```python
from build123d import *

# Parameters (mm, degrees)
EXTRUDE_1_DEPTH     = 2
EXTRUDE_2_DEPTH     = 1.2
SKETCH_4_R          = 1.55
EXTRUDE_3_DEPTH     = 4
EXTRUDE_START       = 3
SKETCH_4_3_R        = 1.55
EXTRUDE_4_DEPTH     = 4
FILLET_1_R          = 3
SKETCH_5_W          = 3.5
SKETCH_5_H          = 2.5
EXTRUDE_5_DEPTH     = 59.375418161
SKETCH_9_W          = 7
SKETCH_9_H          = 4
CUT_EXTRUDE_3_DEPTH = 2
OTHER_START         = -350.004341608
OTHER_1_OUTLINE_W   = 1.5
OTHER_1_OUTLINE_H   = 5.2
OTHER_1_OUTLINE_W_2 = 5.2
OTHER_1_OUTLINE_H_2 = 1.5
OTHER_1_DEPTH       = 1.2
SKETCH_10_R         = 3.4
SKETCH_10_R_2       = 1.4
EXTRUDE_6_DEPTH     = 13.8
EXTRUDE_7_DEPTH     = 2.4
CHAMFER_1_SIZE2     = 1.219331471
CHAMFER_1_SIZE      = 2.5
EXTRUDE_9_DEPTH     = 15.389983971
SKETCH_15_R         = 1.5
CUT_EXTRUDE_4_DEPTH = 407.679532375
FILLET_2_R          = 3
SKETCH_16_R         = 3
CUT_EXTRUDE_5_DEPTH = 408.922716855


# Read off the part's stored shape, not the designer's step: Отступ1
# Some blends are built 0.0001 mm under size
with BuildPart() as part:
    # Эскиз2 → Бобышка-Вытянуть1 (new body)
    with BuildSketch(Plane.XY.offset(0.1)):
        Polygon((-376.904341608, -14.952219826), (-393.804341608, -14.952219826), (-393.804341608, 44.423198335), (-348.804341608, 44.423198335), (-348.804341608, -19.952219826), (-376.904341608, -19.952219826), align=None)
    extrude(amount=EXTRUDE_1_DEPTH)

    # Эскиз3 → Бобышка-Вытянуть2 (add)
    with BuildSketch(Plane(origin=(-348.804341608, 0, 0), x_dir=(0, 0, -1), z_dir=(1, 0, 0))):
        with BuildLine():
            Line((-0.1, -19.952219826), (-0.1, 45.823198335))
            Line((-0.1, 45.823198335), (-58.7849644, 45.823198335))
            ThreePointArc((-58.7849644, 45.823198335), (-79.43775717, 37.268531468), (-87.992424037, 16.615738698))
            Line((-87.992424037, 16.615738698), (-87.992424037, -19.952219826))
            Line((-87.992424037, -19.952219826), (-0.1, -19.952219826))
        make_face()
    extrude(amount=-EXTRUDE_2_DEPTH)

    # Эскиз4 → Бобышка-Вытянуть3 (add)
    with BuildSketch(Plane(origin=(0, -17.952219826, 0), x_dir=(1, 0, 0), z_dir=(0, 1, 0))):
        with BuildLine():
            Line((-357.604341608, -2.1), (-357.604341608, -5.7))
            ThreePointArc((-357.604341608, -5.7), (-356.608504664, -8.104163056), (-354.204341608, -9.1))
            Line((-354.204341608, -9.1), (-350.004341608, -9.1))
            Line((-350.004341608, -9.1), (-350.004341608, -2.1))
            Line((-350.004341608, -2.1), (-357.604341608, -2.1))
        make_face()
        with Locations(Location((-354.204341608, -5.7, 0), (0, 0, 270))):
            Circle(SKETCH_4_R, mode=Mode.SUBTRACT)
    extrude(amount=EXTRUDE_3_DEPTH)

    # Эскиз4<3> → Бобышка-Вытянуть4 (add)
    with BuildSketch(Plane(origin=(0, -17.952219826, 0), x_dir=(1, 0, 0), z_dir=(0, 1, 0)).offset(EXTRUDE_START)):
        with BuildLine():
            Line((-390.304341608, -5.7), (-390.304341608, -2.1))
            Line((-390.304341608, -2.1), (-381.365657691, -2.1))
            Line((-381.365657691, -2.1), (-383.84844185, -7.190461899))
            ThreePointArc((-383.84844185, -7.190461899), (-387.669175192, -9.01285822), (-390.304341608, -5.7))
        make_face()
        with Locations(Location((-386.904341608, -5.7, 0), (0, 0, 180))):
            Circle(SKETCH_4_3_R, mode=Mode.SUBTRACT)
    extrude(amount=EXTRUDE_4_DEPTH)

    # Скругление1
    fillet_1_edges = [part.edges().sort_by_distance(p)[0] for p in [
        (-350.004341608, -18.952219826, 2.1),
        (-350.004341608, 15.235489254, 2.1),
    ]]
    fillet(fillet_1_edges, radius=FILLET_1_R)

    # Эскиз5 → Бобышка-Вытянуть5 (add)
    with BuildSketch(Plane(origin=(0, 44.423198335, 0), x_dir=(1, 0, 0), z_dir=(0, 1, 0))):
        with Locations((-392.054341608, -3.35)):
            Rectangle(SKETCH_5_W, SKETCH_5_H)
    extrude(amount=-EXTRUDE_5_DEPTH)

    # Эскиз9 → Вырез-Вытянуть3 (cut)
    with BuildSketch(Plane(origin=(0, 0, 0.1), x_dir=(-1, 0, 0), z_dir=(0, 0, -1))):
        with Locations((385.390488384, 40.423198335)):
            Rectangle(SKETCH_9_W, SKETCH_9_H)
    extrude(amount=-CUT_EXTRUDE_3_DEPTH, mode=Mode.SUBTRACT)

    # Отступ1 outline → Отступ1 (cut)
    with BuildSketch(Plane.YZ.offset(OTHER_START)):
        with Locations((42.673198335, 13.546937644)):
            Rectangle(OTHER_1_OUTLINE_W, OTHER_1_OUTLINE_H)
        with Locations((42.673198335, 36.546937644)):
            Rectangle(OTHER_1_OUTLINE_W, OTHER_1_OUTLINE_H)
        Polygon((41.843105902, 62.072434127), (41.984560077, 56.874358452), (43.484004983, 56.915162541), (43.342550808, 62.113238216), align=None)
        Polygon((31.397725301, 79.490528515), (35.298941914, 76.052431812), (36.290700579, 77.177782758), (32.389483966, 80.615879461), align=None)
        with Locations((13.847780174, 84.842424037)):
            Rectangle(OTHER_1_OUTLINE_W_2, OTHER_1_OUTLINE_H_2)
        with Locations((-9.152219826, 84.842424037)):
            Rectangle(OTHER_1_OUTLINE_W_2, OTHER_1_OUTLINE_H_2)
    extrude(amount=OTHER_1_DEPTH, mode=Mode.SUBTRACT)

    # Эскиз10 → Бобышка-Вытянуть6 (add)
    # profile 1 of 2: a face of its own
    with BuildSketch(Plane.ZY.offset(350.004341608)):
        with Locations(Location((57.85, 36.323198334, 0), (0, 0, 180))):
            Circle(SKETCH_10_R)
        with Locations(Location((57.85, 36.323198334, 0), (0, 0, 180))):
            Circle(SKETCH_10_R_2, mode=Mode.SUBTRACT)
    # profile 2 of 2: a face of its own
    with BuildSketch(Plane.ZY.offset(350.004341608)):
        with Locations(Location((17.35, 36.323198334, 0), (0, 0, 180))):
            Circle(SKETCH_10_R)
        with Locations(Location((17.35, 36.323198334, 0), (0, 0, 180))):
            Circle(SKETCH_10_R_2, mode=Mode.SUBTRACT)
    extrude(amount=EXTRUDE_6_DEPTH)

    # Эскиз12 → Бобышка-Вытянуть7 (add)
    with BuildSketch(Plane.ZY.offset(350.004341608)):
        with BuildLine():
            Line((77.792424037, 16.615738698), (77.792424037, -19.952219826))
            Line((77.792424037, -19.952219826), (79.792424037, -19.952219826))
            Line((79.792424037, -19.952219826), (79.792424037, 16.615738698))
            ThreePointArc((79.792424037, 16.615738698), (73.639481564, 31.470255863), (58.7849644, 37.623198335))
            Line((58.7849644, 37.623198335), (0.1, 37.623198335))
            Line((0.1, 37.623198335), (0.1, 35.623198335))
            Line((0.1, 35.623198335), (58.7849644, 35.623198335))
            ThreePointArc((58.7849644, 35.623198335), (72.225268002, 30.0560423), (77.792424037, 16.615738698))
        make_face()
    extrude(amount=EXTRUDE_7_DEPTH)

    # Фаска1
    chamfer_1_edges = [part.edges().sort_by_distance(p)[0] for p in [
        (-390.304341608, 16.735489254, 4.6),
    ]]
    chamfer_1_side = [part.faces().sort_by_distance(p)[0] for p in [
        (-390.304341608, 16.735489254, 4.575613371),
    ]]
    chamfer(chamfer_1_edges, length=CHAMFER_1_SIZE - 0.0001, length2=CHAMFER_1_SIZE2 - 0.0001, reference=chamfer_1_side[0])  # a hair under: the kernel refuses the full size

    # Эскиз14 → Бобышка-Вытянуть9 (add)
    with BuildSketch(Plane.ZY.offset(350.004341608)):
        Polygon((77.792424037, -16.979951829), (86.592424037, -16.979951829), (86.592424037, -13.979951829), (81.792424037, -13.979951829), (81.792424037, -4.809951829), (77.792424037, -4.809951829), align=None)
    extrude(amount=EXTRUDE_9_DEPTH)

    # Эскиз15 → Вырез-Вытянуть4 (cut, through all)
    with BuildSketch(Plane(origin=(0, -4.809951829, 0), x_dir=(1, 0, 0), z_dir=(0, 1, 0))):
        with Locations(Location((-357.804325578, -83.692424037, 0), (0, 0, 270))):
            Circle(SKETCH_15_R)
        with BuildLine():
            Line((-363.104325578, -78.236115217), (-363.104325578, -76.736115217))
            Line((-363.104325578, -76.736115217), (-352.504325578, -76.736115217))
            Line((-352.504325578, -76.736115217), (-352.504325578, -78.236115217))
            ThreePointArc((-352.504325578, -78.236115217), (-352.738640153, -78.801800642), (-353.304325578, -79.036115217))
            Line((-353.304325578, -79.036115217), (-354.804325578, -79.036115217))
            ThreePointArc((-354.804325578, -79.036115217), (-354.945746935, -79.09469386), (-355.004325578, -79.236115217))
            Line((-355.004325578, -79.236115217), (-355.004325578, -80.036115217))
            Line((-355.004325578, -80.036115217), (-360.604325578, -80.036115217))
            Line((-360.604325578, -80.036115217), (-360.604325578, -79.236115217))
            ThreePointArc((-360.604325578, -79.236115217), (-360.662904222, -79.09469386), (-360.804325578, -79.036115217))
            Line((-360.804325578, -79.036115217), (-362.304325578, -79.036115217))
            ThreePointArc((-362.304325578, -79.036115217), (-362.870011003, -78.801800642), (-363.104325578, -78.236115217))
        make_face()
    extrude(amount=-CUT_EXTRUDE_4_DEPTH, mode=Mode.SUBTRACT)

    # Скругление2
    # the kernel refuses this fillet: 3 mm, written as the material it adds along each edge
    with BuildSketch(Plane(origin=(-350.004341608, -13.979951829, 81.792424037), x_dir=(0, 1, 0), z_dir=(-1, 0, 0))) as fillet_2_piece_1_section:
        with BuildLine():
            CenterArc((FILLET_2_R, -FILLET_2_R), FILLET_2_R, 90, 90)
            Line((0, -FILLET_2_R), (0, 0))
            Line((0, 0), (FILLET_2_R, 0))
        make_face()
    fillet_2_piece_1 = extrude(amount=15.389983971, mode=Mode.PRIVATE)
    fillet_2_piece_1 = fillet_2_piece_1 - Plane(origin=(-357.804325578, -11.764674138, 83.692424037), x_dir=(0, 0, 1), z_dir=(0, 1, 0)) * Cylinder(1.5, 43, mode=Mode.PRIVATE)
    add(fillet_2_piece_1)

    # Эскиз16 → Вырез-Вытянуть5 (cut, through all)
    with BuildSketch(Plane(origin=(0, -13.979951829, 0), x_dir=(1, 0, 0), z_dir=(0, 1, 0))):
        with Locations((-357.804325578, -83.692424037)):
            Circle(SKETCH_16_R)
    extrude(amount=CUT_EXTRUDE_5_DEPTH, mode=Mode.SUBTRACT)


solid = part.part
```
Verification items for the finished model (mm, model axes). A direction names the side the tool comes from. Give positions to 0.01 mm unless a question says otherwise; leave off trailing zeros. Order: outer loops, then holes, each group sorted by start corner. A loop starts at its lowest first (then second) coordinate and runs counter-clockwise, first axis right, second up. Notation, with made-up numbers: M 54,-20 L 90,-20 A20 ccw 90,12 Z; hole C 82,4.5 d5. An arc over 180 degrees is marked long. Answer in a Markdown table with one row per item. Add a question column.
Item 1: Gauge pin test, flat ends, axial feed: pin 1 (1 mm diameter, centred on x = -349.5, y = 43, fed in from +Z); pin 2 (0.6 mm diameter, centred on y = -16.5, z = 1.5, fed in from -X); pin 3 (1.6 mm diameter, centred on y = -18.5, z = 79, fed in from -X). Record the tip position at first contact, or that the pin passes through.
Item 2: Mould release check, pull along Y, two halves, no side actions. Record for faces 5 (the flat face through (-351, 35.623, 8)), 6 (the cylindrical face through (-356.8, 37.6, 14.2)), 7 (the cylindrical face through (-387.607, -12.98, 9.027)): released by +Y, released by -Y, zero draft, split by the parting line, or undercut.
Item 3: Scan lines: probe 1 along X at (y, z) = (-14, 5); probe 2 along Y at (x, z) = (-350.5, 7.5); probe 3 along X at (y, z) = (-11, 5). Record each from-to range of solid material in increasing order. Write a range as from..to.
Item 4: Section check D-D, the plane x = -378. Enter the section's corners in (y, z), and give its area (3 significant figures).
Item 5: Section check A-A, the plane x = -386.5. Enter the section's corners in (y, z).
Item 6: Tool access check on faces 1 (the flat face through (-388.89, 40, 1)), 2 (the flat face through (-364, -11, 77.792)), 3 (the flat face through (-376.904, -17, 1)), 4 (the flat face through (-390.922, 17.123, 3.368)). Record the directions out of +Z, -Z, +X, -X, +Y, -Y that give a thin tool (end or side, any length) a straight path to the whole face; none if there is none.
Item 7: Section check B-B, the plane z = 29. Enter the section's corners in (x, y).
Filled sheet:
| question | item | result |
|---|---|---|
| 1 | pin 1 | stops at z = 72.32 |
| 1 | pin 2 | stops at x = -376.9 |
| 1 | pin 3 | stops at x = -352.4 |
| 2 | face 5 | undercut |
| 2 | face 6 | split by the parting line |
| 2 | face 7 | zero draft |
| 3 | probe 1 | x = -390.3..-388.29, -385.52..-382.78, -357.6..-355.59, -352.82..-348.8 |
| 3 | probe 2 | y = -17.95..-13.95, 35.62..37.62 |
| 3 | probe 3 | x = -390.3..-388.29, -385.52..-382.78, -350.01..-348.8 |
| 4 | outline | M -14.95,0.1 L 44.42,0.1 L 44.42,2.1 L -14.95,2.1 Z |
| 4 | area | 119 mm^2 |
| 5 | outline | M -14.95,0.1 L 38.42,0.1 L 38.42,2.1 L -10.95,2.1 L -10.95,4.2 L -14.95,4.2 Z; M -14.95,7.2 L -10.95,7.2 L -10.95,9.08 L -14.95,9.08 Z; M 42.42,0.1 L 44.42,0.1 L 44.42,2.1 L 42.42,2.1 Z |
| 6 | face 1 | +Z, -Z |
| 6 | face 2 | -X, +Y, -Y |
| 6 | face 3 | +Z, -Z, -X, -Y |
| 6 | face 4 | +Z, +Y |
| 7 | outline | M -352.4,35.62 L -350,35.62 L -350,-19.95 L -348.8,-19.95 L -348.8,45.82 L -350,45.82 L -350,37.62 L -352.4,37.62 Z |
